Geometry check sheet. Reference: drawing and pictorial views, mm from the part's lowest x, y, z. Give positions to 0.01 mm unless a question says otherwise; leave off trailing zeros. Order: outer loops, then holes, each group sorted by start corner. A loop starts at its lowest first (then second) coordinate and runs counter-clockwise, first axis right, second up.
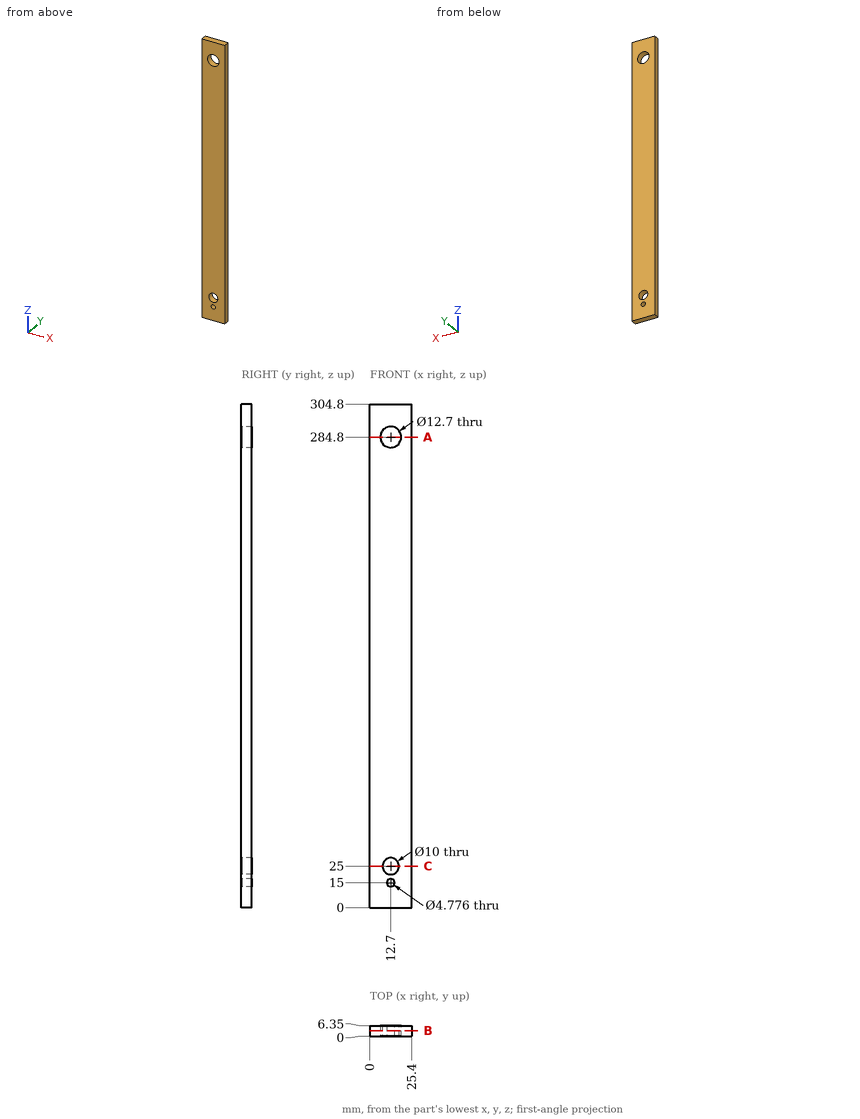
(1) Cross-section at B-B on y = 3.25. Enter the section's corners in (x, z).
Response values:
outline: (0, 0) - (25.4, 0) - (25.4, 304.8) - (0, 304.8) - close; hole circle Ø12.7 at (12.7, 284.8); hole circle Ø10 at (12.7, 25); hole circle Ø4.78 at (12.7, 15)
(2) Cross-section at C-C on z = 25. Enter the section's corners in (x, y).
Response values:
outline: (0, 0) - (7.7, 0) - (7.7, 6.35) - (0, 6.35) - close; (17.7, 0) - (25.4, 0) - (25.4, 6.35) - (17.7, 6.35) - close
(3) Cross-section at A-A on z = 284.8. Enter the section's corners in (x, y), then the cut area to 3 significant figures.
Response values:
outline: (0, 0) - (6.35, 0) - (6.35, 6.35) - (0, 6.35) - close; (19.05, 0) - (25.4, 0) - (25.4, 6.35) - (19.05, 6.35) - close
area: 80.6 mm2
(4) Material ranges on L1, parallel to Z at x = 12.7, y = 2; L2, parallel to Z at x = 11.25, y = 4.5; L3, parallel to Z at x = 18, y = 4.75, recorded low to high.
Response values:
L1: z = 0 to 12.61, 17.39 to 20, 30 to 278.45, 291.15 to 304.8
L2: z = 0 to 13.1, 16.9 to 20.21, 29.79 to 278.62, 290.98 to 304.8
L3: z = 0 to 281.3, 288.3 to 304.8
(5) Gauge pin test, flat end, axial feed: pin 1 Ø9 at (x, z) = (12.7, 25) entering from -Y. Record the tip position at first contact, or that the pin passes through.
Response values:
pin 1: passes through
